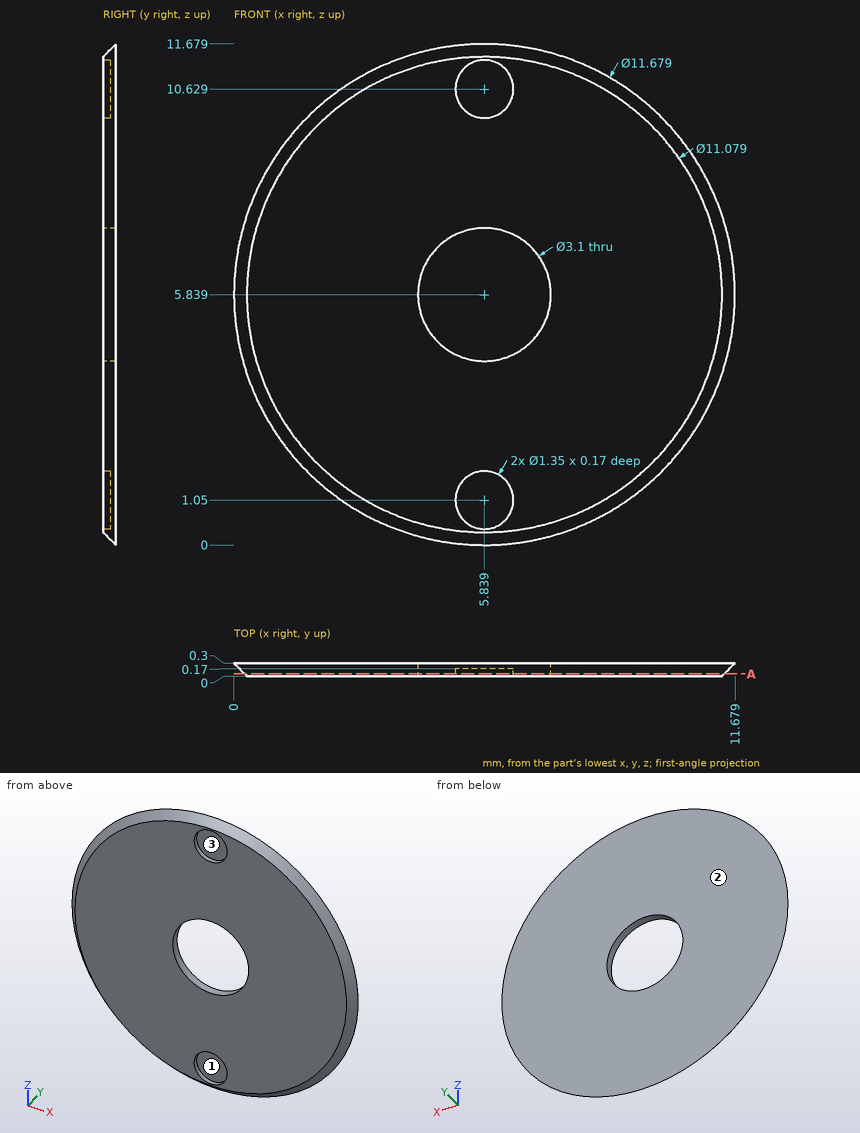
The drawing under review shows one solid part. Ordinate dimensions are in mm from its lowest x, y, z. Coordinates: 2 decimals unless noted, no trailing zeros. Use CSV: the item, a comma, the result in double quotes. Start each with the question number.
1. Add section A-A on y = 0.05. Count the separate pieces of the cut face and the enclosed holes in it.
2. Mouldability with a two-part tool opening along Z and no side actions: class the marked faces 1, 2 and 3 as released by +Z, released by -Z, zero draft, split by the parting line, or undercut.
3. Clearance check with a flat-ended pin moving along its axis: pin 1 (0.7 mm diameter, centred on x = 6, z = 1, fed in from -Y). State where the tip first meets the part, or that it passes through.
4. To check wall thickness, follow probe 1 along Z at (x, y) = (6.25, 0.1) (1 decimal); probe 2 along Z at (x, y) = (4.5, 0.15); probe 3 along X at (y, z) = (0.05, 4.75) (1 decimal). State the ranges of each line that lie inside material, in increasing order.
Resolved:
1,separate pieces,"1"
1,enclosed holes,"3"
2,face 1,"undercut"
2,face 2,"zero draft"
2,face 3,"undercut"
3,pin 1,"y = 0.17"
4,probe 1,"0.2 to 0.5, 1.6 to 4.3, 7.3 to 10.1, 11.2 to 11.5"
4,probe 2,"0.31 to 5.06, 6.62 to 11.37"
4,probe 3,"0.4 to 4.7, 6.9 to 11.3"
